Input: part model. Units: mm. Frame: model coordinates. Face numbers are marked on the shaded views. A direction names the side the tool comes from. Round coordinates to 2 decimals unless told otherwise and drop trailing zeros. One line per item, written item: value. Start each with the question number.
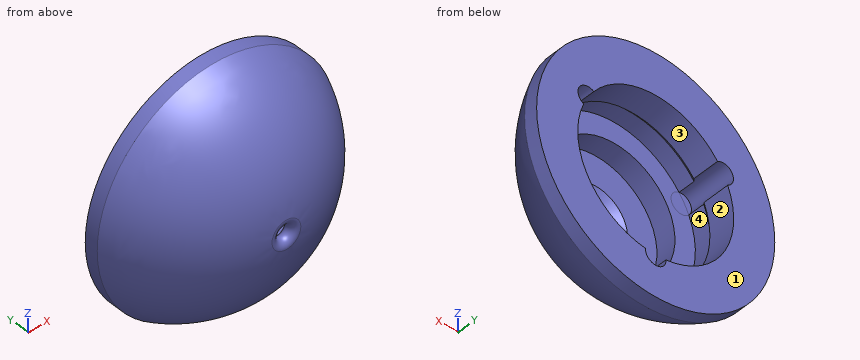
Autodesk Inventor part; units mm, degrees
ref_plane "YZ Plane" through (0, 0, 0) normal (1, 0, 0) x (0, 1, 0)
ref_plane "XZ Plane" through (0, 0, 0) normal (0, 1, 0) x (-1, 0, 0)
ref_plane "XY Plane" through (0, 0, 0) normal (0, 0, 1) x (1, 0, 0)
sketch "Sketch1" plane through (0, 0, 0) normal (0, 0, 1) x (1, 0, 0)
  line L0 (-35.8694, 36.1667) -> (26.1213, 35.095) construction
  line L1 (26.1213, 35.095) -> (24.9917, -30.2436) construction
  line L2 (24.9917, -30.2436) -> (-36.999, -29.1719) construction
  line L3 (-36.999, -29.1719) -> (-35.8694, 36.1667) construction
  line L4 (0, -29.8115) -> (0, 35.5466) construction
  line L5 (-17.5, 14) -> (17.5, 14)
  line L6 (17.5, 14) -> (17.5, 12)
  arc A0 (0, 0.1813) -> (17.5, 12) centre (-0.0907, 19.1811) ccw
  arc A1 (1.5, 2.169) -> (2.1161, 0.3097) centre (2, 1.3029) ccw
  line L7 (12, 7) -> (12, 9.5)
  line L8 (12, 9.5) -> (11, 10.5)
  line L9 (11, 10.5) -> (11, 14)
  line L10 (4.6714, 4) -> (9, 4)
  line L11 (9, 4) -> (9, 7)
  line L12 (9, 7) -> (12, 7)
  line L13 (1.5, 2.169) -> (4.6714, 4)
  line L14 (1.5, 2.169) -> (0, 1.3029)
  point P0 (0, 0)
  point P1 (0, 14)
  point P2 (0, 0)
  dimension "d3" = 26.1213
  dimension "d7" = 24.9955
  dimension "d9" = 35
  dimension "d10" = 62
  dimension "d18" = 21.5466
  dimension "d19" = 14
  dimension "d26" = 19
  dimension "d27" = 1
  dimension "d34" = 22
  dimension "d38" = 135
  dimension "d39" = 2
  dimension "d41" = 2
  dimension "d44" = 24
  dimension "d54" = 11.831
  dimension "d82" = 18
  dimension "d83" = 10
  dimension "d86" = 7
  dimension "d87" = 3.5
  dimension "d90" = 150
revolve "Revolution1" add sketch "Sketch1" angle 360 about axis through (0, -29.8115, 0) along (0, 1, 0)
sketch "Sketch2" plane through (0, 14, 0) normal (0, 1, 0) x (1, 0, 0)
  circle A0 centre (0, 0) radius 11
  point P0 (0, 0)
hole "Hole1" at (0, 14, 0) direction (0, -1, 0) diameter 22.9175 depth 5
sketch "Sketch3" plane through (0, 14, 0) normal (0, 1, 0) x (1, 0, 0)
  circle A0 centre (0, 0) radius 11.4587
  point P0 (0, 0)
  point P1 (0, 11.4587)
hole "Hole2" at (0, 14, -11.4587) direction (0, -1, 0) diameter 3 depth 7
pattern_circular "Circular Pattern1" count 3 over 360 about axis through (0, 13, 0) along (0, -1, 0) of "Hole2"
equation "\"d3\" = 0.421311 * d10"
equation "\"d7\" = 0.403153 * d10"
equation "\"d18\" = 0.347525 * d10"
properties part number "015" material "Stainless Steel, Austenitic"
Item 1: Line query: L1, parallel to Y at x = 12, z = 2; L2, parallel to X at y = 9, z = 6.5; L3, parallel to X at y = 9.25, z = -12. Output: solid intervals per line, ascending.
Item 2: Pull-direction query (X, two-part tool) for the marked faces 1 and 2; classes: released by +X, released by -X, zero draft, split by the parting line, or undercut.
Item 3: Reachability of the marked faces 3 and 4 from +Z, -Z, +X, -X, +Y, -Y: full face, straight path, thin tool, end or side. Return the list, or none.
Item 4: First-contact query: pin 1 Ø1.5 at (y, z) = (3, 3) entering from +X; pin 2 Ø3 at (y, z) = (5, 0.5) entering from -X; pin 3 Ø2 at (y, z) = (5.5, 10) entering from -X. Flat tips, straight axial feed; report the tip coordinate or a pass-through.
Geometry results:
1. L1: y = 4.66 to 14
1. L2: x = -14.57 to -11.21, 11.21 to 14.57
1. L3: x = -10.74 to -1.4, 1.4 to 10.74
2. face 1: zero draft
2. face 2: undercut
3. face 3: +Y
3. face 4: none
4. pin 1: stops at x = 10.6
4. pin 2: stops at x = -14.05
4. pin 3: stops at x = -10.21
